The listing builds one solid part. Answer for the finished solid, in the listing's coordinates (mm). Face numbers are marked on the shaded views. Give positions to 0.01 mm unless a question says otherwise; leave off trailing zeros. Loops run counter-clockwise (first coordinate to the right, second up) from the corner with the lowest first, then second, coordinate; pieces in that order, holes last.
Item 1: The mould has two halves that part along X. Classify the marked faces 1 and 2: pulls with the +X half, pulls with the -X half, needs draft (parallel to the pull), parting line crosses it, or undercut.
Item 2: Consider line 1 along Y through (x, z) = (45, 4); line 2 along Y through (x, z) = (62.5, 9.5). Determine where each line is inside the solid, lowest interval first.
Item 3: Section D-D, the plane x = 16 is taken. Give the vertices of the cut face in (y, z).
Item 4: This flat-tipped pin is pushed along its axis until it touches: pin 1 Ø3 at (y, z) = (5.5, 4) entering from -X. Where does it stop, or does it pass through?
Item 5: Section A-A, the plane x = 135 is taken. Give the vertices of the cut face in (y, z).
Item 6: Section B-B, the plane y = 5 is taken. Give the number of separate pieces and of enclosed holes in the cut face, and give its area (3 significant figures).
Autodesk Fusion 360 part; units mm, degrees
sketch "Sketch1" plane through (0, 0, 0) normal (0, 0, 1) x (1, 0, 0)
  line L0 (0, 0) -> (150, 0)
  line L1 (150, 0) -> (150, 10)
  line L2 (150, 10) -> (0, 10)
  line L3 (0, 10) -> (0, 0)
  dimension "d1" = 150
  dimension "d2" = 10
extrude "Extrude1" add sketch "Sketch1" along normal blind 10
sketch "Sketch2" plane through (0, 0, 0) normal (1, 0, 0) x (0, 1, 0)
  circle A0 centre (5, 5) radius 4
  circle A1 centre (5, 5) radius 3.5
  dimension "d5" = 8
  dimension "d6" = 7
extrude "Extrude2" add sketch "Sketch2" against normal blind 3
sketch "Sketch3" plane through (150, 0, 0) normal (1, 0, 0) x (0, 1, 0)
  line L0 (0, 0) -> (10, 0)
  line L1 (10, 0) -> (10, 10)
  line L2 (10, 10) -> (0, 10)
  line L3 (0, 10) -> (0, 0)
  circle A0 centre (5, 5) radius 4.5
  dimension "d9" = 9
extrude "Extrude3" cut sketch "Sketch3" against normal blind 3 contours A0
fillet "Fillet1" radius 0.25 1 edges at (150, 0.8045, 6.6273)
sketch "Sketch4" plane through (0, 0, 0) normal (0, 0, -1) x (1, 0, 0)
  line L0 (0, 0) -> (0, -10)
  line L1 (0, -10) -> (150, -10)
  line L2 (150, -10) -> (150, 0)
  line L3 (150, 0) -> (0, 0)
  circle A0 centre (5, -5) radius 4.5
  circle A1 centre (25, -5) radius 4.5
  circle A2 centre (65, -5) radius 4.5
  circle A3 centre (45, -5) radius 4.5
  circle A4 centre (145, -5) radius 4.5
  circle A5 centre (125, -5) radius 4.5
  circle A6 centre (105, -5) radius 4.5
  circle A7 centre (85, -5) radius 4.5
  dimension "d14" = 9
  dimension "d15" = 9
  dimension "d16" = 9
  dimension "d17" = 9
  dimension "d18" = 9
  dimension "d19" = 9
  dimension "d20" = 9
  dimension "d21" = 9
extrude "Extrude4" cut sketch "Sketch4" against normal blind 30 contours A0 | A1 | A2 | A3 | A4 | A5 | A6 | A7
sketch "Sketch5" plane through (0, 10, 0) normal (0, 1, 0) x (-1, 0, 0)
  line L0 (-150, 0) -> (0, 0)
  line L1 (0, 0) -> (0, 10)
  line L2 (0, 10) -> (-150, 10)
  line L3 (-150, 10) -> (-150, 0)
  circle A0 centre (-15, 5) radius 4.5
  circle A1 centre (-35, 5) radius 4.5
  circle A2 centre (-75, 5) radius 4.5
  circle A3 centre (-55, 5) radius 4.5
  circle A4 centre (-95, 5) radius 4.5
  circle A5 centre (-115, 5) radius 4.5
  circle A6 centre (-135, 5) radius 4.5
  dimension "d24" = 9
  dimension "d25" = 9
  dimension "d26" = 9
  dimension "d27" = 9
  dimension "d28" = 9
  dimension "d29" = 9
  dimension "d30" = 9
extrude "Extrude5" cut sketch "Sketch5" against normal blind 30 contours A0 | A1 | A2 | A3 | A4 | A5 | A6
sketch "Sketch6" plane through (0, 0, 0) normal (0, 0, -1) x (1, 0, 0)
  line L0 (0, 0) -> (0, -10)
  line L1 (0, -10) -> (150, -10)
  line L2 (150, -10) -> (150, 0)
  line L3 (150, 0) -> (0, 0)
  circle A0 centre (145, -5) radius 4.5
  circle A1 centre (65, -5) radius 4.5
  circle A2 centre (5, -5) radius 4.5
  circle A3 centre (85, -5) radius 4.5
  circle A4 centre (125, -5) radius 4.5
  circle A5 centre (45, -5) radius 4.5
  circle A6 centre (25, -5) radius 4.5
  circle A7 centre (105, -5) radius 4.5
extrude "Extrude6" add sketch "Sketch6" against normal blind 10 contours A0
sketch "Sketch7" plane through (150, 0, 0) normal (1, 0, 0) x (0, 1, 0)
  line L0 (0, 0) -> (10, 0)
  line L1 (10, 0) -> (10, 10)
  line L2 (10, 10) -> (0, 10)
  line L3 (0, 10) -> (0, 0)
  circle A0 centre (5, 5) radius 4.75
extrude "Extrude7" cut sketch "Sketch7" against normal blind 3 contours A0
extrude "Extrude8" cut 1 faces at (147, 4.6477, 2.9844) along direction (-1, 0, 0) blind 0.5
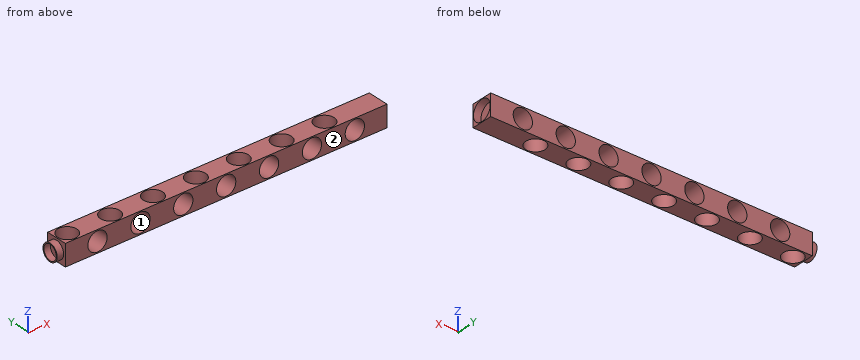
Worked answers:
1. face 1: undercut
1. face 2: needs draft
2. line 1: y = 0 to 0.5, 9.5 to 10
2. line 2: y = 0 to 1.26, 8.74 to 10
3. outline: (0, 0) - (10, 0) - (10, 0.61) - (0, 0.61) - close; (0, 9.39) - (10, 9.39) - (10, 10) - (0, 10) - close
4. pin 1: stops at x = 0
5. outline: (0, 0) - (10, 0) - (10, 0.5) - (0, 0.5) - close; (0, 9.5) - (10, 9.5) - (10, 10) - (0, 10) - close
6. separate pieces: 8
6. enclosed holes: 7
6. area: 394 mm2
